Here's how the part is built. I have some questions about the finished solid (model axes, mm). Face numbers are marked on the shaded views. Give positions to 0.01 mm unless a question says otherwise; leave off trailing zeros. Loops run counter-clockwise (first coordinate to the right, second up) from the corner with the lowest first, then second, coordinate; pieces in that order, holes last.
Q1. If we section it at D-D (x = 11): Please give me the cut outline in (y, z), plus the area to 3 significant figures.
Q2. We'd pull the mould along Y, two halves only. Please class the marked faces 1, 2 and 3: +Y half, -Y half, draft (parallel to the pull), parting line (faces both ways), or undercut.
Q3. If we section it at A-A (y = 0): Please give me the cut outline in (x, z).
Q4. If we section it at B-B (z = 0): Please give me the cut outline in (x, y).
Q5. I need wall thicknesses on line 1 (Y direction, x = 8.25, z = 0); line 2 (Y direction, x = 6, z = 7); line 3 (Z direction, x = 7, y = 3.5). Which ranges of each line are inside material? Lowest first, please.
Q6. Will these pins go through, and if not, where does the flat tip stop? P1, Ø3, axis at x = 7, z = 4.5, coming from the +Y side; P2, Ø1.5, axis at x = 10, y = -10, coming from the +Z side; P3, Ø4, axis at x = 2.5, y = -4.5, coming from the -Z side.
Q7. If we section it at C-C (z = -3): Please give me the cut outline in (x, y).
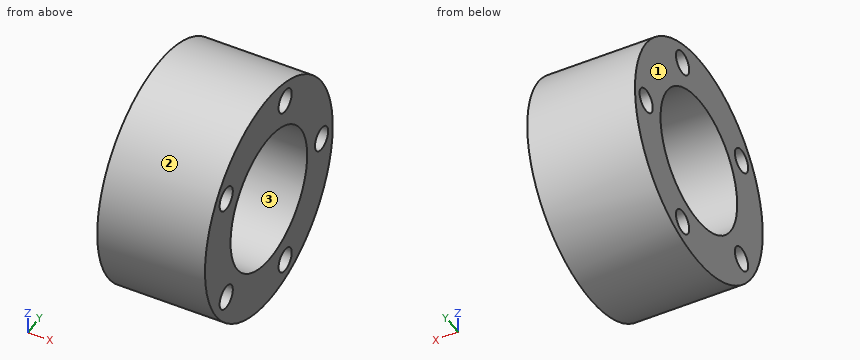
from build123d import *

# Parameters (mm, degrees)
SKETCH1_R           = 13.543461356
SKETCH1_R_2         = 8.128
BOSS_EXTRUDE1_DEPTH = 12.7
SKETCH2_R           = 1.397
CUT_EXTRUDE1_DEPTH  = 13.7


with BuildPart() as part:
    # Sketch1 → Boss-Extrude1 (new body)
    with BuildSketch(Plane(origin=(0, 0, 0), x_dir=(0, 0, -1), z_dir=(1, 0, 0))):
        Circle(SKETCH1_R)
        Circle(SKETCH1_R_2, mode=Mode.SUBTRACT)
    extrude(amount=BOSS_EXTRUDE1_DEPTH)

    # Sketch2 → Cut-Extrude1 (cut, through all)
    with BuildSketch(Plane.ZY):
        with Locations((0, 11.176)):
            Circle(SKETCH2_R)
        with Locations((10.629007626, 3.453573929)):
            Circle(SKETCH2_R)
        with Locations((6.56908798, -9.041573929)):
            Circle(SKETCH2_R)
        with Locations((-6.56908798, -9.041573929)):
            Circle(SKETCH2_R)
        with Locations((-10.629007626, 3.453573929)):
            Circle(SKETCH2_R)
    extrude(amount=-CUT_EXTRUDE1_DEPTH, mode=Mode.SUBTRACT)


solid = part.part
Check sheet entries:
1. outline: circle Ø27.09 at (0, 0); hole circle Ø2.79 at (-9.04, -6.57); hole circle Ø2.79 at (-9.04, 6.57); hole circle Ø16.26 at (0, 0); hole circle Ø2.79 at (3.45, -10.63); hole circle Ø2.79 at (3.45, 10.63); hole circle Ø2.79 at (11.18, 0)
1. area: 338 mm2
2. face 1: draft
2. face 2: parting line
2. face 3: undercut
3. outline: (0, -13.54) - (12.7, -13.54) - (12.7, -8.13) - (0, -8.13) - close; (0, 8.13) - (12.7, 8.13) - (12.7, 13.54) - (0, 13.54) - close
4. outline: (0, -13.54) - (12.7, -13.54) - (12.7, -8.13) - (0, -8.13) - close; (0, 8.13) - (12.7, 8.13) - (12.7, 9.78) - (0, 9.78) - close; (0, 12.57) - (12.7, 12.57) - (12.7, 13.54) - (0, 13.54) - close
5. line 1: y = -13.54 to -8.13, 8.13 to 9.78, 12.57 to 13.54
5. line 2: y = -11.59 to -10.37, -7.71 to -4.13, 4.13 to 11.59
5. line 3: z = -13.08 to -12.03, -9.23 to -7.34, 7.34 to 9.23, 12.03 to 13.08
6. P1: stops at y = 13.21
6. P2: stops at z = 9.89
6. P3: stops at z = -13.31
7. outline: (0, -13.21) - (12.7, -13.21) - (12.7, -7.55) - (0, -7.55) - close; (0, 7.55) - (12.7, 7.55) - (12.7, 13.21) - (0, 13.21) - close
